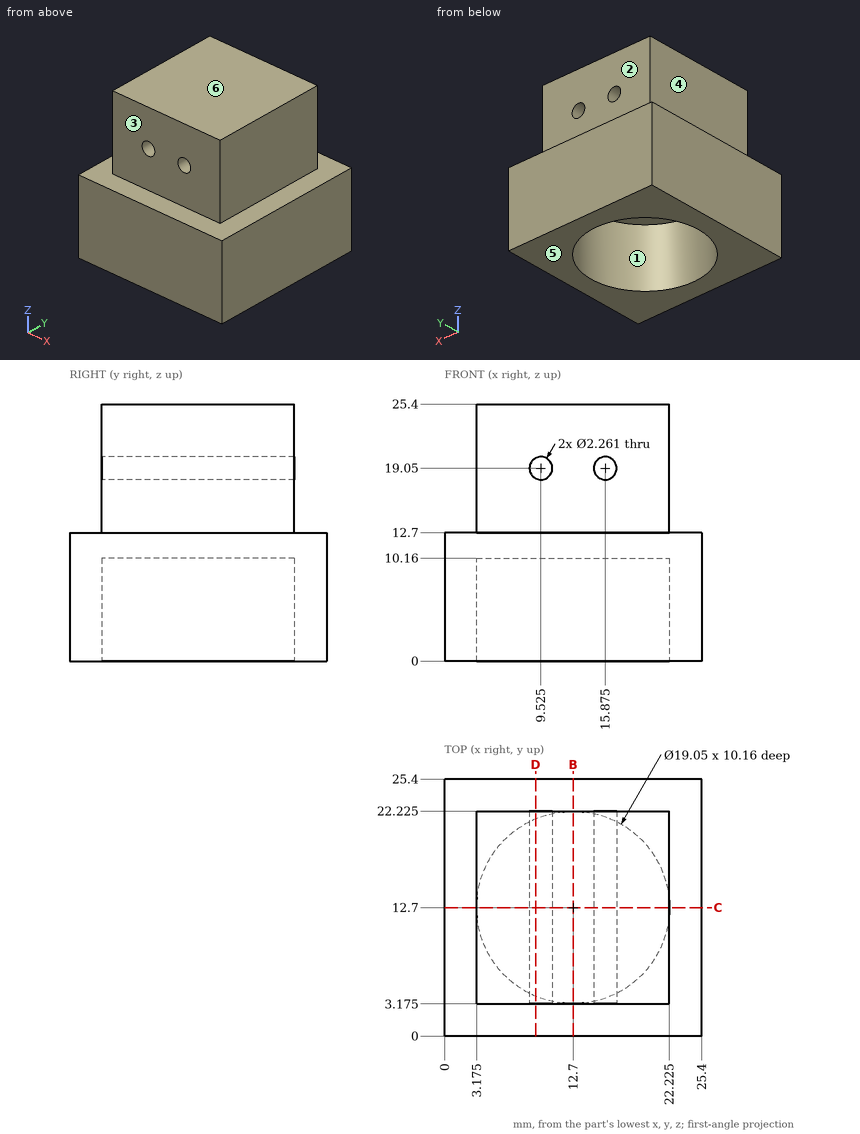
Drawing for the job (mm, zero at the part's lowest x, y, z). A direction names the side the tool comes from. Round coordinates to 2 decimals unless told otherwise and drop trailing zeros. Order: outer loops, then holes, each group sorted by start corner. A loop starts at its lowest first (then second) coordinate and runs counter-clockwise, first axis right, second up. Notation, with made-up numbers: (-18, 18.5) -> (26, 18.5) arc R32 cw to (26, 49.5) -> close; hole circle Ø3 at (-17, -33). An arc over 180 degrees is marked (long way). Put each result on its own line as item: value.
Q1. Wall check: line 1 (X direction, y = 8.5, z = 19.05) (1 decimal); line 2 (Y direction, x = 12.7, z = 3) (1 decimal); line 3 (X direction, y = 16.5, z = 20.75) (1 decimal). Give the ranges that are in metal, low to high. Write a range as [from, to].
From the geometry:
line 1: x = [3.2, 8.4], [10.7, 14.7], [17, 22.2]
line 2: y = [0, 3.2], [22.2, 25.4]
line 3: x = [3.2, 22.2]
Q2. Band-saw the part on D-D (x = 9). Give the cut face in (y, z) (1 decimal).
From the geometry:
outline: (0, 0) -> (3.9, 0) -> (3.9, 10.2) -> (21.5, 10.2) -> (21.5, 0) -> (25.4, 0) -> (25.4, 12.7) -> (22.2, 12.7) -> (22.2, 18) -> (3.2, 18) -> (3.2, 12.7) -> (0, 12.7) -> close; (3.2, 20.1) -> (22.2, 20.1) -> (22.2, 25.4) -> (3.2, 25.4) -> close
Q3. Pin check, flat tips, straight feed: pin 1 Ø4 at (x, z) = (20.5, 18) entering from -Y (3 decimals); pin 2 Ø5.5 at (x, y) = (9.5, 12) entering from -Z; pin 3 Ø6.5 at (y, z) = (16.5, 18.5) entering from -X (3 decimals). Stop position of each tip, or through.
From the geometry:
pin 1: stops at y = 3.175
pin 2: stops at z = 10.16
pin 3: stops at x = 3.175
Q4. Tool access for the marked faces 1, 2 and 3: list every direction of +Z, -Z, +X, -X, +Y, -Y with a clear straight run to the whole face (end or side of a thin tool).
From the geometry:
face 1: -Z
face 2: +Z, +X, -X, +Y
face 3: +Z, +X, -X, -Y
Q5. Band-saw the part on B-B (x = 12.7). Give the cut face in (y, z) (1 decimal).
From the geometry:
outline: (0, 0) -> (3.2, 0) -> (3.2, 10.2) -> (22.2, 10.2) -> (22.2, 0) -> (25.4, 0) -> (25.4, 12.7) -> (22.2, 12.7) -> (22.2, 25.4) -> (3.2, 25.4) -> (3.2, 12.7) -> (0, 12.7) -> close
Q6. Pull direction Z, two halves, no side cores. Call the marked faces 4, 5 and 6: pulls with the +Z half, pulls with the -Z half, needs draft (parallel to the pull), parting line crosses it, or undercut.
From the geometry:
face 4: needs draft
face 5: pulls with the -Z half
face 6: pulls with the +Z half
Q7. Band-saw the part on C-C (y = 12.7). State how many separate pieces and enclosed holes the cut face has, and give its area (3 significant figures).
From the geometry:
separate pieces: 1
enclosed holes: 2
area: 363 mm2
